Can you work these out from the model? Positions are in its coordinate system, mm. A direction names the side the tool comes from. Give positions to 0.01 mm unless a question says otherwise; leave off trailing zeros. Order: outer loops, then holes, each group sorted by start corner. A loop starts at its lowest first (then second) coordinate and runs counter-clockwise, first axis right, second up. Notation, with made-up numbers: M -15.5,62.25 L 14.5,62.25 A8 ccw 14.5,67.25 Z; hole C 69.25,14 d6. An arc over 180 degrees is marked long. Use one line per item in the form item = value. Start each with the question number.
1. I want a section at C-C, the plane x = 152.5. List the corners of the cut face in (y, z) for me.
2. I want a section at A-A, the plane y = 57.5. List the corners of the cut face in (x, z) for me, and give its area (3 significant figures).
3. I want a section at D-D, the plane y = 12.5. List the corners of the cut face in (x, z) for me.
4. I want a section at B-B, the plane z = 34. List the corners of the cut face in (x, y) for me.
5. Will these pins go through, and if not, where does the flat tip stop? P1, Ø5, axis at y = 7, z = 121.5, coming from the -X side; P2, Ø9, axis at x = 31.5, z = 130.2, coming from the +Y side; P3, Ø8, axis at x = 108, z = 86.04, coming from the -Y side.
6. I need wall thicknesses on L1, parallel to Y at x = 152.5, z = 23.5; L2, parallel to Z at x = 57, y = 9.25; L3, parallel to Y at x = 152, z = 14. Which ranges of each line are inside material? Lowest first, please.
7. We'd pull the mould along Y, two halves only. Please class faces 1 (the face through (97, 25, 95.407)), 2 (the face through (84, 70, 49)), 3 (the face through (72.5, 30, 48)): +Y half, -Y half, draft (parallel to the pull), parting line (faces both ways), or undercut.
8. For faces 4 (the face through (126.111, 50.28, 104.147)), 5 (the face through (106, 15, 88)), 6 (the face through (52.225, 25.07, 113.049)), 7 (the face through (9.5, 35.5, 30)), which set-ups out of +Z, -Z, +X, -X, +Y, -Y let a thin tool reach every point of the face, with its end or its side?
Autodesk Inventor part; units mm, degrees
ref_plane "YZ Plane" through (0, 0, 0) normal (1, 0, 0) x (0, 1, 0)
ref_plane "XZ Plane" through (0, 0, 0) normal (0, 1, 0) x (-1, 0, 0)
ref_plane "XY Plane" through (0, 0, 0) normal (0, 0, 1) x (1, 0, 0)
sketch "Sketch24" plane through (0, 0, 0) normal (0, 0, 1) x (1, 0, 0)
  line L0 (0, 0) -> (165, 0)
  line L1 (165, 0) -> (165, 70)
  line L2 (165, 70) -> (0, 70)
  line L3 (0, 70) -> (0, 0)
  circle A0 centre (12.5, 57.5) radius 2.5
  circle A1 centre (12.5, 35) radius 2.5
  circle A2 centre (12.5, 12.5) radius 2.5
  line L4 (12.5, 57.5) -> (12.5, 12.5) construction
  line L5 (82.5, 70) -> (82.5, 0) construction
  circle A3 centre (152.5, 57.5) radius 2.5
  circle A4 centre (152.5, 35) radius 2.5
  circle A5 centre (152.5, 12.5) radius 2.5
  line L6 (152.5, 57.5) -> (152.5, 12.5) construction
  point P0 (0, 35)
  dimension "d100" = 165
  dimension "d101" = 70
  dimension "d102" = 5
  dimension "d103" = 5
  dimension "d104" = 5
  dimension "d105" = 45
  dimension "d106" = 12.5
extrude "Extrusion21" add sketch "Sketch24" along normal blind 30
sketch "Sketch25" plane through (0, 0, 30) normal (0, 0, 1) x (1, 0, 0)
  line L0 (165, 70) -> (0, 70)
  line L1 (0, 0) -> (165, 0)
  line L2 (25, 70) -> (140, 70)
  line L3 (140, 70) -> (140, 0)
  line L4 (140, 0) -> (25, 0)
  line L5 (25, 0) -> (25, 70)
  point P0 (82.5, 70)
  dimension "d109" = 115
extrude "Extrusion22" add sketch "Sketch25" along normal blind 150
sketch "Sketch26" plane through (0, 70, 0) normal (0, 1, 0) x (1, 0, 0)
  line L0 (25, -30) -> (25, -180)
  line L1 (25, -130.2035) -> (53.75, -80.4071)
  line L2 (53.75, -80.4071) -> (111.25, -80.4071)
  line L3 (111.25, -80.4071) -> (140, -130.2035)
  line L4 (140, -130.2035) -> (111.25, -180)
  line L5 (111.25, -180) -> (53.75, -180)
  line L6 (53.75, -180) -> (25, -130.2035)
  line L7 (140, -30) -> (140, -180)
  line L8 (140, -180) -> (25, -180)
  point P0 (0, 0)
  point P1 (82.5, -130.2035)
  point P2 (82.5, -180)
extrude "Extrusion23" cut sketch "Sketch26" against normal through all contours L6 L8 L0 | L4 L7 L8
sketch "Sketch27" plane through (0, 70, 0) normal (0, 1, 0) x (1, 0, 0)
  line L0 (25, -130.2035) -> (53.75, -180)
  line L1 (111.25, -180) -> (53.75, -180)
  line L2 (111.25, -180) -> (140, -130.2035)
  line L3 (53.75, -180) -> (25, -130.2035)
  line L4 (25, -130.2035) -> (53.75, -80.4071)
  line L5 (53.75, -80.4071) -> (111.25, -80.4071)
  line L6 (111.25, -80.4071) -> (140, -130.2035)
  line L7 (140, -130.2035) -> (111.25, -180)
  line L8 (111.25, -180) -> (53.75, -180)
  line L9 (53.1726, -79.4071) -> (23.8453, -130.2035)
  line L10 (23.8453, -130.2035) -> (53.1726, -181)
  line L11 (53.1726, -181) -> (111.8274, -181)
  line L12 (111.8274, -181) -> (141.1547, -130.2035)
  line L13 (141.1547, -130.2035) -> (111.8274, -79.4071)
  line L14 (111.8274, -79.4071) -> (53.1726, -79.4071)
  point P0 (0, 0)
  point P1 (82.5, -130.2035)
  dimension "d114" = 1
extrude "Extrusion24" cut sketch "Sketch27" against normal blind 40 contours L4 L5 L6 L2 L1 L0 | L14 L13 L12 L11 L10 L9
sketch "Sketch28" plane through (0, 30, 0) normal (0, 1, 0) x (1, 0, 0)
  circle A0 centre (31.5, -130.2035) radius 2.5
  line L0 (53.75, -180) -> (25, -130.2035)
  line L1 (140, -128.2035) -> (140, -130.2035) construction
  line L2 (25, -130.2035) -> (140, -130.2035) construction
  circle A1 centre (82.5, -130.2035) radius 2.5 construction
  circle A2 centre (133.5, -130.2035) radius 2.5 construction
  line L3 (31.5, -130.2035) -> (133.5, -130.2035) construction
  circle A3 centre (57, -174.3708) radius 2.5
  circle A4 centre (108, -174.3708) radius 2.5
  circle A5 centre (133.5, -130.2035) radius 2.5
  circle A6 centre (108, -86.0362) radius 2.5
  circle A7 centre (57, -86.0362) radius 2.5
  point P0 (0, 0)
  dimension "d117" = 5
  dimension "d118" = 5
  dimension "d119" = 5
  dimension "d120" = 102
  dimension "d123" = 360
extrude "Extrusion25" cut sketch "Sketch28" against normal through all
sketch "Sketch29" plane through (0, 0, 0) normal (0, -1, 0) x (1, 0, 0)
  circle A0 centre (57, 174.3708) radius 2.5 construction
  circle A1 centre (108, 86.0362) radius 2.5 construction
  line L0 (57, 174.3708) -> (108, 86.0362) construction
  circle A2 centre (57, 174.3708) radius 7.5
  line L1 (31.5, 130.2035) -> (133.5, 130.2035) construction
  circle A3 centre (31.5, 130.2035) radius 7.5
  line L2 (57, 86.0362) -> (108, 174.3708) construction
  circle A4 centre (57, 86.0362) radius 7.5
  line L3 (108, 86.0362) -> (57, 174.3708) construction
  circle A5 centre (108, 86.0362) radius 7.5
  line L4 (133.5, 130.2035) -> (31.5, 130.2035) construction
  circle A6 centre (133.5, 130.2035) radius 7.5
  line L5 (108, 174.3708) -> (57, 86.0362) construction
  circle A7 centre (108, 174.3708) radius 7.5
  point P0 (0, 0)
  point P1 (82.5, 130.2035)
  point P2 (82.5, 130.2035)
  point P3 (82.5, 130.2035)
  point P4 (82.5, 130.2035)
  point P5 (82.5, 130.2035)
  point P6 (82.5, 130.2035)
  dimension "d127" = 15
  dimension "d130" = 360
extrude "Extrusion26" cut sketch "Sketch29" against normal blind 15
sketch "Sketch30" plane through (0, 30, 0) normal (0, 1, 0) x (1, 0, 0)
  line L0 (53.75, -180) -> (25, -130.2035) construction
  line L1 (111.25, -180) -> (53.75, -180) construction
  line L2 (140, -130.2035) -> (111.25, -180) construction
  circle A0 centre (133.5, -130.2035) radius 2.5 construction
  circle A1 centre (31.5, -130.2035) radius 2.5 construction
  circle A2 centre (133.5, -130.2035) radius 2.5 construction
  line L3 (31.5, -130.2035) -> (133.5, -130.2035) construction
  line L4 (102.5897, -165) -> (62.4103, -165)
  line L5 (62.4103, -165) -> (42.3205, -130.2035)
  line L6 (42.3205, -130.2035) -> (62.4103, -95.4071)
  line L7 (62.4103, -95.4071) -> (102.5897, -95.4071)
  line L8 (102.5897, -95.4071) -> (122.6795, -130.2035)
  line L9 (122.6795, -130.2035) -> (102.5897, -165)
  point P0 (0, 0)
  point P1 (82.5, -130.2035)
  point P2 (82.5, -130.2035)
  dimension "d134" = 15
extrude "Extrusion27" cut sketch "Sketch30" against normal blind 10
sketch "Sketch31" plane through (62.4103, 30, 95.4071) normal (0, 0, 1) x (1, 0, 0)
  line L0 (-9.2376, 40) -> (49.4171, 40)
  line L1 (-9.2376, 40) -> (-9.2376, 0)
  line L2 (-9.2376, 0) -> (49.4171, 0)
  line L3 (49.4171, 40) -> (49.4171, 0)
  line L4 (0, 0) -> (40.1795, 0)
  line L5 (0, 0) -> (0, -10)
  line L6 (0, -10) -> (40.1795, -10)
  line L7 (40.1795, 0) -> (40.1795, -10)
  line L8 (10.0897, -10) -> (30.0897, -10)
  line L9 (30.0897, -10) -> (30.0897, 10)
  line L10 (30.0897, 10) -> (10.0897, 10)
  line L11 (10.0897, 10) -> (10.0897, -10)
  point P0 (-62.4103, -30)
  point P1 (20.0897, -10)
  dimension "d137" = 20
  dimension "d138" = 20
extrude "Extrusion28" cut sketch "Sketch31" against normal through all contours L11 L10 L9 L2 | L2 L9 L6 L11
sketch "Sketch32" plane through (25, 0, 30) normal (-1, 0, 0) x (0, 0, 1)
  circle A0 centre (65.4071, 65) radius 2.5
  line L0 (0, 70) -> (98.2035, 70)
  point P0 (-30, 0)
  point P1 (49.4071, 70)
  dimension "d141" = 5
  dimension "d142" = 5
  dimension "d143" = 16
extrude "Extrusion29" cut sketch "Sketch32" against normal through all
properties part number "TARM01" material "ABS Plastic"
Check result:
q1.outline = M 0,0 L 10,0 L 10,30 L 0,30 Z; M 15,0 L 32.5,0 L 32.5,30 L 15,30 Z; M 37.5,0 L 55,0 L 55,30 L 37.5,30 Z; M 60,0 L 70,0 L 70,30 L 60,30 Z
q2.outline = M 0,0 L 10,0 L 10,30 L 0,30 Z; M 15,0 L 150,0 L 150,30 L 140,30 L 140,128.2 L 111.83,79.41 L 53.17,79.41 L 25,128.2 L 25,30 L 15,30 Z; M 155,0 L 165,0 L 165,30 L 155,30 Z
q2.area = 11,700 mm2
q3.outline = M 0,0 L 10,0 L 10,30 L 0,30 Z; M 15,0 L 150,0 L 150,30 L 140,30 L 140,126.46 A7.5 cw long 135.9,137.31 L 115.35,172.89 A7.5 cw long 103.04,180 L 61.96,180 A7.5 cw long 49.65,172.89 L 29.1,137.31 A7.5 cw long 25,126.46 L 25,30 L 15,30 Z; M 155,0 L 165,0 L 165,30 L 155,30 Z; hole C 57,86.04 d15; hole C 108,86.04 d15
q4.outline = M 25,0 L 140,0 L 140,70 L 25,70 Z; hole M 72.5,20 L 92.5,20 L 92.5,40 L 72.5,40 Z
q5.P1 = 25
q5.P2 = 30
q5.P3 = 15
q6.L1 = 0 to 10, 15 to 32.5, 37.5 to 55, 60 to 70
q6.L2 = 0 to 78.54, 93.54 to 166.87
q6.L3 = 0 to 10.05, 14.95 to 32.55, 37.45 to 55.05, 59.95 to 70
q7.face_1 = draft
q7.face_2 = +Y half
q7.face_3 = undercut
q8.face_4 = +Z, +Y
q8.face_5 = -Y
q8.face_6 = +Y
q8.face_7 = +Z, -X, +Y, -Y
